Geometry: final body of the model. Coordinates: model frame, mm. A direction names the side the tool comes from. Give positions to 0.01 mm unless a question says otherwise; leave off trailing zeros. Write each loop counter-clockwise with the first axis right and the second up, starting at its lowest first coordinate (ties: lowest second). Pieces come first, ordered by that corner, then holes.
Autodesk Inventor part; units mm, degrees
ref_plane "YZ Plane" through (0, 0, 0) normal (1, 0, 0) x (0, 1, 0)
ref_plane "XZ Plane" through (0, 0, 0) normal (0, 1, 0) x (-1, 0, 0)
ref_plane "XY Plane" through (0, 0, 0) normal (0, 0, 1) x (1, 0, 0)
sketch "Sketch1" plane through (0, 0, 0) normal (0, 0, 1) x (1, 0, 0)
  line L0 (0, 0) -> (50.8, 0)
  line L1 (50.8, 0) -> (50.8, 50.8)
  line L2 (50.8, 50.8) -> (47.625, 50.8)
  line L3 (44.45, 47.625) -> (44.45, 12.7)
  line L4 (38.1, 6.35) -> (3.175, 6.35)
  line L5 (0, 3.175) -> (0, 0)
  arc A0 (3.175, 6.35) -> (0, 3.175) centre (3.175, 3.175) ccw
  arc A1 (47.625, 50.8) -> (44.45, 47.625) centre (47.625, 47.625) ccw
  arc A2 (38.1, 6.35) -> (44.45, 12.7) centre (38.1, 12.7) ccw
  dimension "d0" = 50.8
  dimension "d1" = 6.35
  dimension "d2" = 3.175
  dimension "d3" = 6.35
extrude "Extrusion1" add sketch "Sketch1" along normal blind 177.8
sketch "Sketch2" plane through (0, 0, 0) normal (0, -1, 0) x (1, 0, 0)
  line L0 (0, 0) -> (50.8, 0)
  line L1 (0, 177.8) -> (50.8, 177.8)
  line L2 (0, 0) -> (0, 177.8)
  point P0 (12.7, 165.1)
  point P1 (31.75, 165.1)
  point P2 (12.7, 12.7)
  point P3 (31.75, 12.7)
  dimension "d6" = 19.05
  dimension "d7" = 12.7
  dimension "d8" = 12.7
  dimension "d9" = 12.7
hole "Hole1" at (12.7, 0, 165.1) at (31.75, 0, 165.1) at (12.7, 0, 12.7) at (31.75, 0, 12.7) direction (0, 1, 0) diameter 6.35 end through all
sketch "Sketch3" plane through (50.8, 0, 0) normal (1, 0, 0) x (0, 0, -1)
  line L0 (0, 0) -> (0, 50.8)
  line L1 (0, 50.8) -> (-177.8, 50.8)
  line L2 (-177.8, 0) -> (-177.8, 50.8)
  point P0 (-165.1, 19.05)
  point P1 (-165.1, 38.1)
  point P2 (-12.7, 19.05)
  point P3 (-12.7, 38.1)
  dimension "d17" = 19.05
  dimension "d18" = 12.7
  dimension "d19" = 12.7
  dimension "d20" = 12.7
hole "Hole2" at (50.8, 19.05, 165.1) at (50.8, 38.1, 165.1) at (50.8, 19.05, 12.7) at (50.8, 38.1, 12.7) direction (-1, 0, 0) diameter 6.35 end through all
properties part number "Right Angle" material "Aluminum 6061"
Q1. Section C-C on z = 165.1. Output: boundary loops of the cut face in (x, y) (3 decimals).
Filled sheet:
outline: (0, 0) - (9.525, 0) - (9.525, 6.35) - (3.175, 6.35) arc R3.175 ccw to (0, 3.175) - close; (15.875, 0) - (28.575, 0) - (28.575, 6.35) - (15.875, 6.35) - close; (34.925, 0) - (50.8, 0) - (50.8, 15.875) - (44.45, 15.875) - (44.45, 12.7) arc R6.35 cw to (38.1, 6.35) - (34.925, 6.35) - close; (44.45, 22.225) - (50.8, 22.225) - (50.8, 34.925) - (44.45, 34.925) - close; (44.45, 41.275) - (50.8, 41.275) - (50.8, 50.8) - (47.625, 50.8) arc R3.175 ccw to (44.45, 47.625) - close
Q2. Section A-A on x = 31.75. Output: boundary loops of the cut face in (y, z) (3 decimals), plus the area to 3 significant figures.
Filled sheet:
outline: (0, 0) - (6.35, 0) - (6.35, 9.525) - (0, 9.525) - close; (0, 15.875) - (6.35, 15.875) - (6.35, 161.925) - (0, 161.925) - close; (0, 168.275) - (6.35, 168.275) - (6.35, 177.8) - (0, 177.8) - close
area: 1,050 mm2
Q3. Ray query, line 1 along Z through (x, y) = (31.75, 3.5) (3 decimals); line 2 along X through (y, z) = (2, 12.7) (3 decimals); line 3 along Y through (x, z) = (48.5, 168). Return the intervals inside material, ascending.
Filled sheet:
line 1: z = 0 to 9.525, 15.875 to 161.925, 168.275 to 177.8
line 2: x = 0 to 9.525, 15.875 to 28.575, 34.925 to 50.8
line 3: y = 0 to 17.76, 20.34 to 36.81, 39.39 to 50.8
Q4. Access query for faces 1 (the flat face through (49, 50.8, 88)), 2 (the flat face through (44.45, 30, 88)). Directions: +Z, -Z, +X, -X, +Y, -Y. A direction counts if a zero-diameter tool reaches every point of the face in a straight line with its end or side. Return the directions, or none.
Filled sheet:
face 1: +Z, -Z, +X, -X, +Y
face 2: +Z, -Z, -X, +Y
Q5. Pull-direction query (Z, two-part tool) for faces 3 (the flat face through (37, 5, 177.8)), 4 (the cylindrical face through (47.58, 39.32, 162.17)), 5 (the cylindrical face through (32.97, 3.22, 162.17)), 6 (the flat face through (21, 6.35, 88)); classes: released by +Z, released by -Z, zero draft, split by the parting line, or undercut.
Filled sheet:
face 3: released by +Z
face 4: undercut
face 5: undercut
face 6: zero draft
Q6. Pin query (flat end, axial travel): P1, Ø7.5, axis at x = 12.7, z = 165.1, coming from the +Y side; P2, Ø3, axis at y = 10, z = 157.5, coming from the -X side; P3, Ø10, axis at y = 19.05, z = 12.7, coming from the -X side. Return the tip coordinate at first contact, or that it passes through.
Filled sheet:
P1: stops at y = 6.35
P2: stops at x = 42.86
P3: stops at x = 44.45
Q7. Section B-B on y = 19.05. Output: boundary loops of the cut face in (x, z) (3 decimals).
Filled sheet:
outline: (44.45, 0) - (50.8, 0) - (50.8, 9.525) - (44.45, 9.525) - close; (44.45, 15.875) - (50.8, 15.875) - (50.8, 161.925) - (44.45, 161.925) - close; (44.45, 168.275) - (50.8, 168.275) - (50.8, 177.8) - (44.45, 177.8) - close
Q8. Section D-D on z = 92.5. Output: boundary loops of the cut face in (x, y) (3 decimals).
Filled sheet:
outline: (0, 0) - (50.8, 0) - (50.8, 50.8) - (47.625, 50.8) arc R3.175 ccw to (44.45, 47.625) - (44.45, 12.7) arc R6.35 cw to (38.1, 6.35) - (3.175, 6.35) arc R3.175 ccw to (0, 3.175) - close
